The figure shows three views and two pictorial views of one solid part (mm, origin at its lowest corner). Answer the questions. A direction names the side the tool comes from. Coordinates: 2 decimals unless noted, no trailing zeros. Loops run counter-clockwise (first coordinate to the right, second up) from the corner with the lowest first, then second, coordinate; pieces in that order, holes last.
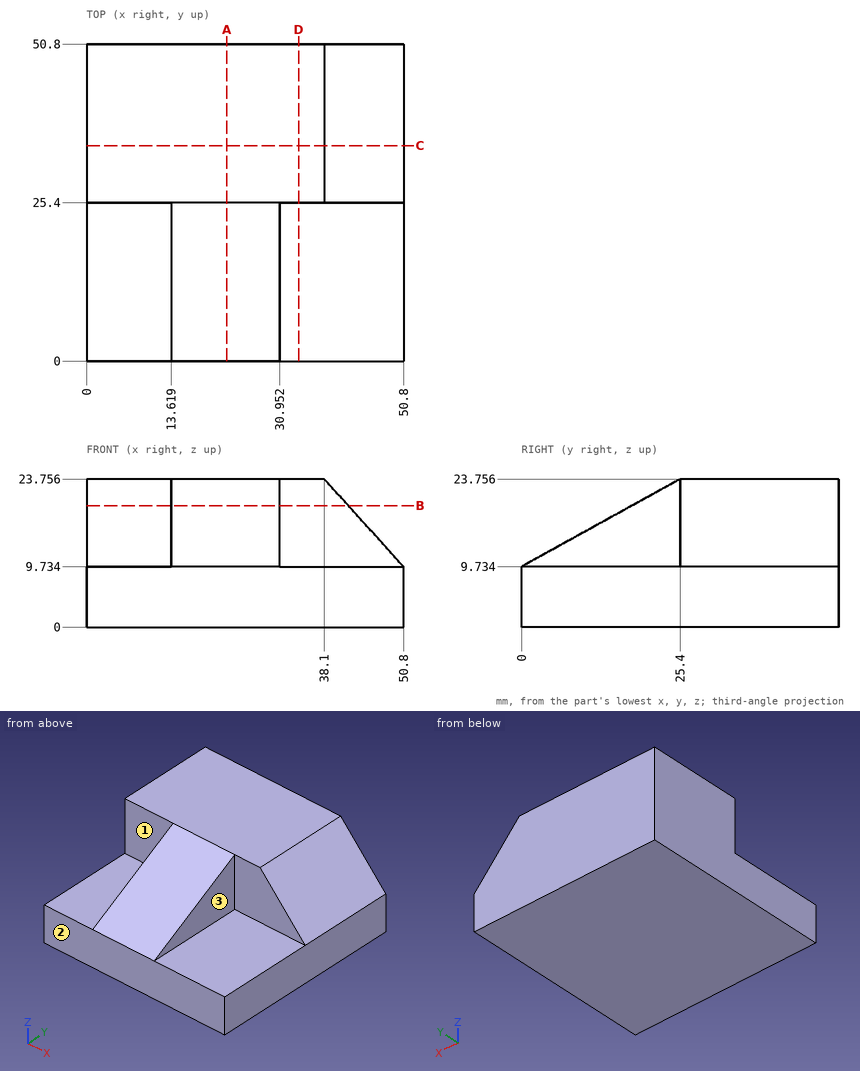
1. Straight lines are drawn through the part: probe 1 along Y at (x, z) = (44, 10.5); probe 2 along Z at (x, y) = (48.5, 7.5); probe 3 along X at (y, z) = (9, 12.25). For each, find the intervals that lie inside material, in ascending order.
2. A cutting plane is placed at D-D, the plane x = 34. Give the vertices of the cut face in (y, z), then the cut area to 3 significant figures.
3. Each of these flat-tipped pins is pushed along its axis until it touches: P1, Ø10, axis at x = 19.5, y = 20, coming from the +Z side (1 decimal); P2, Ø4, axis at x = 45, z = 19, coming from the -Y side; P3, Ø1.5, axis at x = 26.5, y = 14, coming from the +Z side. Where does it stop, or does it pass through?
4. A cutting plane is placed at A-A, the plane x = 22.5. Give the vertices of the cut face in (y, z).
5. A cutting plane is placed at B-B, the plane z = 19.5. Give the vertices of the cut face in (x, y) (1 decimal).
6. A cutting plane is placed at C-C, the plane y = 34.5. Give the vertices of the cut face in (x, z), then the cut area to 3 significant figures.
7. For the marked faces 1, 2 and 3, determine the directions among +Z, -Z, +X, -X, +Y, -Y from which every point of the face is accessible in a straight line to the end or side of a thin tool.
Answers below:
1. probe 1: y = 25.4 to 50.8
1. probe 2: z = 0 to 9.73
1. probe 3: x = 13.62 to 30.95
2. outline: (0, 0) - (50.8, 0) - (50.8, 23.76) - (25.4, 23.76) - (25.4, 9.73) - (0, 9.73) - close
2. area: 851 mm2
3. P1: stops at z = 23.5
3. P2: stops at y = 25.4
3. P3: stops at z = 17.88
4. outline: (0, 0) - (50.8, 0) - (50.8, 23.76) - (25.4, 23.76) - (0, 9.73) - close
5. outline: (0, 25.4) - (13.6, 25.4) - (13.6, 17.7) - (31, 17.7) - (31, 25.4) - (42, 25.4) - (42, 50.8) - (0, 50.8) - close
6. outline: (0, 0) - (50.8, 0) - (50.8, 9.73) - (38.1, 23.76) - (0, 23.76) - close
6. area: 1,120 mm2
7. face 1: +Z, -X, -Y
7. face 2: +Z, -Z, +X, -X, -Y
7. face 3: +Z, +X, -Y
